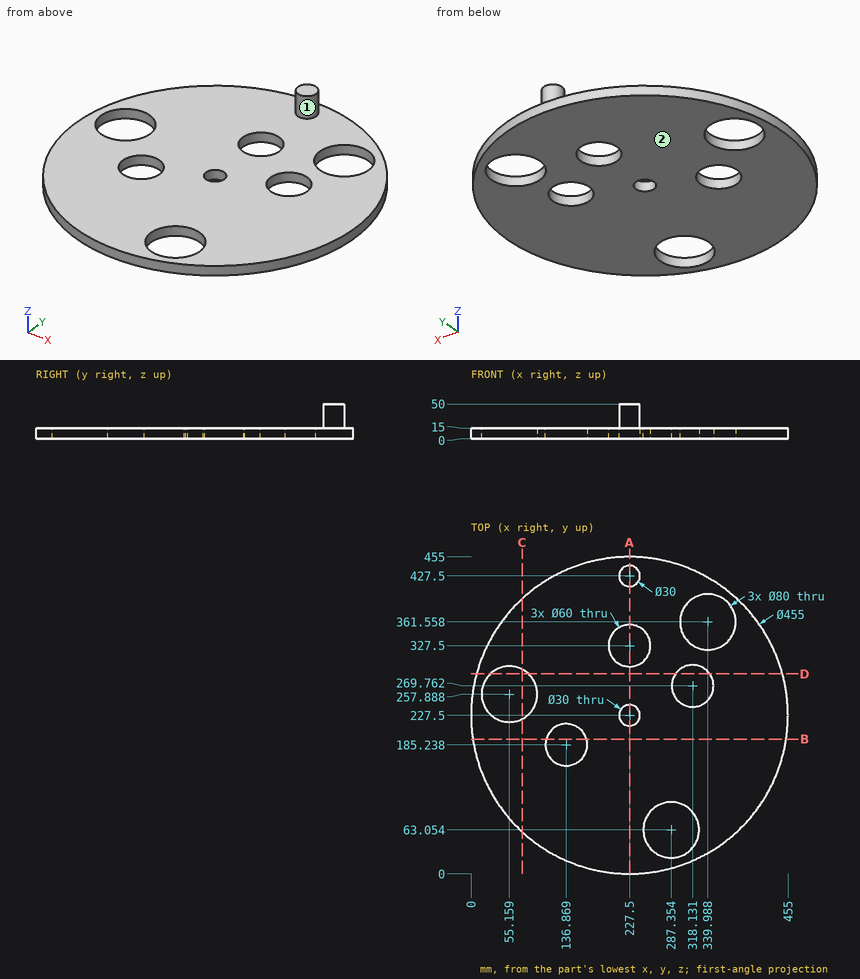
Verification items for this drawing (mm, ordinates from the low corner). A direction names the side the tool comes from. Round coordinates to 2 decimals unless told otherwise and drop trailing zeros. Write each loop counter-clockwise with the first axis right and the second up, starting at its lowest first coordinate (ties: lowest second). Pieces come first, ordered by that corner, then holes. Notation, with made-up numbers: (79.5, 72) - (108.5, 72) arc R14 cw to (108.5, 98) - close; hole circle Ø6 at (-0.75, 88). An arc over 180 degrees is marked (long way). Answer as a JSON object with one key per item and string values. Group by question number.
Q1. Go/stop test with flat-tipped pins: pin 1 Ø5 at (x, z) = (118, 10.5) entering from +Y; pin 2 Ø3 at (y, z) = (218, 8.5) entering from -X; pin 3 Ø2 at (x, z) = (218.5, 37.5) entering from -Y. Record where each tip stops, or that it passes through.
Q2. Tool access check on the marked faces 1 and 2. Record the directions out of +Z, -Z, +X, -X, +Y, -Y that give a thin tool (end or side, any length) a straight path to the whole face; none if there is none.
Q3. Section check C-C, the plane x = 73.5. Enter the section's corners in (y, z) (1 decimal).
Q4. Thickness scan on line 1 (X direction, y = 248, z = 5) (1 decimal); line 2 (Z direction, x = 201.5, y = 60.5); line 3 (X direction, y = 162.5, z = 14) (1 decimal). Record the ranges inside material, lowest first.
Q5. Section check A-A, the plane x = 227.5. Enter the section's corners in (y, z).
Q6. Section check D-D, the plane y = 287. Enter the section's corners in (x, z).
Q7. Section check B-B, the plane y = 193.5. Enter the section's corners in (x, z) (1 decimal), plus the area to 3 significant figures.
Found:
{
 "1": {"pin 1": "stops at y = 428.27", "pin 2": "stops at x = 0.14", "pin 3": "stops at y = 414.81"},
 "2": {"face 1": "+Z", "face 2": "-Z, +X, -X, +Y, -Y"},
 "3": {"outline": "(60, 0) - (222.3, 0) - (222.3, 15) - (60, 15) - close; (293.4, 0) - (395, 0) - (395, 15) - (293.4, 15) - close"},
 "4": {"line 1": "x = 0.9 to 16.4, 93.9 to 297.5, 338.8 to 454.1", "line 2": "z = 0 to 15", "line 3": "x = 9.5 to 117.3, 156.4 to 445.5"},
 "5": {"outline": "(0, 0) - (212.5, 0) - (212.5, 15) - (0, 15) - close; (242.5, 0) - (297.5, 0) - (297.5, 15) - (242.5, 15) - close; (357.5, 0) - (455, 0) - (455, 15) - (442.5, 15) - (442.5, 50) - (412.5, 50) - (412.5, 15) - (357.5, 15) - close"},
 "6": {"outline": "(7.92, 0) - (27.73, 0) - (27.73, 15) - (7.92, 15) - close; (82.59, 0) - (293.58, 0) - (293.58, 15) - (82.59, 15) - close; (342.68, 0) - (447.08, 0) - (447.08, 15) - (342.68, 15) - close"},
 "7": {"outline": "(2.6, 0) - (108, 0) - (108, 15) - (2.6, 15) - close; (165.7, 0) - (452.4, 0) - (452.4, 15) - (165.7, 15) - close", "area": "5,880 mm^2"}
}
